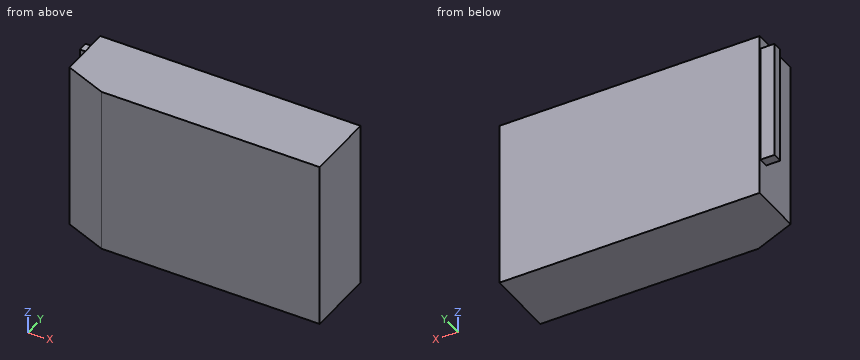
```python
from build123d import *

# Parameters (mm, degrees)
BOX041_W                  = 41
BOX041_H                  = 12
BOX041_DEPTH              = 200
BOX041_PLACEMENT_ANGLE    = 22
BOX_W                     = 186
BOX_H                     = 50
BOX_DEPTH                 = 120
BOX039_W                  = 11
BOX039_H                  = 7
BOX039_DEPTH              = 85
FUSION012_PLACEMENT_ANGLE = 180


with BuildPart() as cube036:
    # Box041 → Box041 (new body)
    with BuildSketch(Plane.XY):
        with Locations((20.5, 6)):
            Rectangle(BOX041_W, BOX041_H)
    extrude(amount=BOX041_DEPTH)


with BuildPart() as cube036_1:
    # Box041 placement: moved
    add(cube036.part.moved(Location((-1.797588, 37.123258, -8))).rotate(Axis((-1.797588, 37.123258, -8), (0, 0, 1)), BOX041_PLACEMENT_ANGLE))


with BuildPart() as cut012:
    # Box → Box (new body)
    with BuildSketch(Plane.XY):
        with Locations((93, 25)):
            Rectangle(BOX_W, BOX_H)
    extrude(amount=BOX_DEPTH)

    # Cut012: cut Cube036
    add(cube036_1.part, mode=Mode.SUBTRACT)


with BuildPart() as obj1:
    # Box039 → Box039 (new body)
    with BuildSketch(Plane(origin=(-10, 1, 9), x_dir=(1, 0, 0), z_dir=(0, 0, 1))):
        with Locations((5.5, 3.5)):
            Rectangle(BOX039_W, BOX039_H)
    extrude(amount=BOX039_DEPTH)

    # Fusion012: union Cut012
    add(cut012.part)


with BuildPart() as obj1_1:
    # Fusion012 placement: moved
    add(obj1.part.moved(Location((0, -65.5, 174))).rotate(Axis((0, -65.5, 174), (1, 0, 0)), FUSION012_PLACEMENT_ANGLE))


solid = obj1_1.part
```
Model file for the job. Use its own axes, mm. Give positions to 0.01 mm unless a question says otherwise; leave off trailing zeros. Write each loop counter-clockwise with the first axis right and the second up, starting at its lowest first coordinate (ties: lowest second). Pieces come first, ordered by that corner, then holes. Notation, with made-up numbers: (-16, 26.25) -> (3, 26.25) arc R9 ccw to (3, 42.25) -> close; hole circle Ø8 at (43, 14.25). An arc over 180 degrees is marked (long way). Use CSV: the item, a comma, the result in double quotes. Start each with the question number.
1) Pin check, flat tips, straight feed: P1, Ø5.5, axis at x = -6, y = -70.5, coming from the -Z side; P2, Ø3, axis at y = -82.5, z = 140.5, coming from the -X side; P3, Ø5, axis at x = -3, z = 141, coming from the -Y side. Stop position of each tip, or through.
2) Cut at A-A on z = 136. List the corners of the cut face in (x, y).
3) Drill centre lines: L1, parallel to X at y = -76, z = 147.5; L2, parallel to Y at x = 26.5, z = 138.5; L3, parallel to X at y = -111, z = 145.5. Where is each one in solid material? Low to high.
4) Cut at C-C on y = -84.5. List the corners of the cut face in (x, z), plus the area to 3 significant figures.
5) Cut at B-B on x = 13.5. List the corners of the cut face in (y, z), plus the area to 3 significant figures.
6) Cut at D-D on z = 73.5. List the corners of the cut face in (x, y), plus the area to 3 significant figures.
Final values:
1,P1,"stops at z = 80"
1,P2,"stops at x = 0"
1,P3,"stops at y = -73.5"
2,outline,"(-10, -73.5) -> (0, -73.5) -> (0, -103.35) -> (30.07, -115.5) -> (186, -115.5) -> (186, -65.5) -> (0, -65.5) -> (0, -66.5) -> (-10, -66.5) -> close"
3,L1,"x = 0 to 186"
3,L2,"y = -114.06 to -65.5"
3,L3,"x = 18.94 to 186"
4,outline,"(0, 54) -> (186, 54) -> (186, 174) -> (0, 174) -> close"
4,area,"22,300 mm2"
5,outline,"(-108.8, 54) -> (-65.5, 54) -> (-65.5, 174) -> (-108.8, 174) -> close"
5,area,"5,200 mm2"
6,outline,"(0, -103.35) -> (30.07, -115.5) -> (186, -115.5) -> (186, -65.5) -> (0, -65.5) -> close"
6,area,"9,120 mm2"
